Read the model definition and answer for the solid it produces. Units are mm, in the model's axes. Coordinates: 2 decimals unless noted, no trailing zeros. Write each loop counter-clockwise with the first axis right and the second up, starting at its lowest first coordinate (ties: lowest second). Pieces come first, ordered by that corner, then holes. Notation, with made-up numbers: (12, 7) -> (53, 7) arc R36 cw to (53, 44) -> close; hole circle Ø10 at (-2, 77). An arc over 180 degrees is marked (long way). Write item = value, one per line. Start each with the question number.
1) Flat-ended cylindrical pins translate along their axes: pin 1 Ø4 at (x, z) = (215.5, 6.5) entering from +Y; pin 2 Ø5 at (x, z) = (-51.5, 6) entering from -Y; pin 3 Ø4.5 at (y, z) = (-214, 5) entering from +X; pin 4 Ø5 at (x, z) = (-85, 9) entering from +Y. Find the tip coordinate at first contact, or state that the pin passes through.
2) Find the intervals of material crossed by line 1 along Y through (x, z) = (28, 5); line 2 along Y through (x, z) = (-43, 5.5), in increasing order. Write a range as from..to.
3) Section C-C (y = -120) is taken. Determine the outline of the cut face in (x, z), plus the area to 3 significant figures.
4) Section A-A (x = 87.5) is taken. Count the separate pieces of the cut face and the enclosed holes in it, plus the area to 3 significant figures.
from build123d import *

# Parameters (mm, degrees)
SKETCH_1_W             = 420
SKETCH_1_H             = 420
EXTRUDE_1_DEPTH        = 10
SKETCH_2_W             = 200
SKETCH_2_H             = 8
EXTRUDE_2_DEPTH        = 8
CUT_EXTRUDE_1_REACH    = 381.109
SKETCH_3_R             = 2
FILLET_1_R             = 4
FILLET_1_OF_MIRROR_1_R = 4
SKETCH_4_W             = 8
SKETCH_4_H             = 200
EXTRUDE_3_DEPTH        = 8
FILLET_2_R             = 4
CUT_EXTRUDE_2_REACH    = 387.679
SKETCH_5_R             = 2
FILLET_2_OF_MIRROR_3_R = 4


with BuildPart() as part:
    # 草图1 → 凸台-拉伸1 (new body)
    with BuildSketch(Plane.XY):
        Rectangle(SKETCH_1_W, SKETCH_1_H)
    extrude_1 = extrude(amount=EXTRUDE_1_DEPTH)

    # 草图2 → 凸台-拉伸2 (add)
    with BuildSketch(Plane(origin=(0, 210, 0), x_dir=(1, 0, 0), z_dir=(0, 1, 0))):
        with Locations((0, -5)):
            Rectangle(SKETCH_2_W, SKETCH_2_H)
    extrude_2 = extrude(amount=EXTRUDE_2_DEPTH)

    # 草图3 → 切除-拉伸1 (cut, up to next)
    with BuildSketch(Plane(origin=(100, 0, 0), x_dir=(0, 0, -1), z_dir=(1, 0, 0)), mode=Mode.PRIVATE) as cut_extrude_1_sk1:
        with Locations((-5, 214)):
            Circle(SKETCH_3_R)
    cut_extrude_1_tool1 = extrude(cut_extrude_1_sk1.sketch, amount=-CUT_EXTRUDE_1_REACH, mode=Mode.PRIVATE) & part.part
    cut_extrude_1 = cut_extrude_1_tool1.solids().sort_by_distance((100, 214, 5))[0]
    add(cut_extrude_1, mode=Mode.SUBTRACT)

    # 圆角1
    fillet_1_edges = [part.edges().sort_by_distance(p)[0] for p in [
        (0, 218, 1),
        (0, 218, 9),
    ]]
    fillet(fillet_1_edges, radius=FILLET_1_R - 0.0001)  # a hair under: the kernel refuses the full size

    # 镜向1: 凸台-拉伸1, 凸台-拉伸2, 切除-拉伸1 across plane
    add(extrude_1.mirror(Plane.ZX))
    add(extrude_2.mirror(Plane.ZX))
    add(cut_extrude_1.mirror(Plane.ZX), mode=Mode.SUBTRACT)

    # 圆角1 of 镜向1
    fillet_1_of_mirror_1_edges = [part.edges().sort_by_distance(p)[0] for p in [
        (0, -218, 1),
        (0, -218, 9),
    ]]
    fillet(fillet_1_of_mirror_1_edges, radius=FILLET_1_OF_MIRROR_1_R - 0.0001)  # a hair under: the kernel refuses the full size

    # 草图4 → 凸台-拉伸3 (add)
    with BuildSketch(Plane.ZY.offset(210)):
        with Locations((5, 0)):
            Rectangle(SKETCH_4_W, SKETCH_4_H)
    extrude_3 = extrude(amount=EXTRUDE_3_DEPTH)

    # 圆角2
    fillet_2_edges = [part.edges().sort_by_distance(p)[0] for p in [
        (-218, 0, 9),
        (-218, 0, 1),
    ]]
    fillet(fillet_2_edges, radius=FILLET_2_R - 0.0001)  # a hair under: the kernel refuses the full size

    # 草图5 → 切除-拉伸2 (cut, up to next)
    with BuildSketch(Plane.XZ.offset(100), mode=Mode.PRIVATE) as cut_extrude_2_sk1:
        with Locations(Location((-214, 5, 0), (0, 0, 270))):
            Circle(SKETCH_5_R)
    cut_extrude_2_tool1 = extrude(cut_extrude_2_sk1.sketch, amount=-CUT_EXTRUDE_2_REACH, mode=Mode.PRIVATE) & part.part
    cut_extrude_2 = cut_extrude_2_tool1.solids().sort_by_distance((-214, -100, 5))[0]
    add(cut_extrude_2, mode=Mode.SUBTRACT)

    # 镜向3: 凸台-拉伸3, 切除-拉伸2 across plane
    add(extrude_3.mirror(Plane(origin=(0, 0, 0), x_dir=(0, 0, 1), z_dir=(1, 0, 0))))
    add(cut_extrude_2.mirror(Plane(origin=(0, 0, 0), x_dir=(0, 0, 1), z_dir=(1, 0, 0))), mode=Mode.SUBTRACT)

    # 圆角2 of 镜向3
    fillet_2_of_mirror_3_edges = [part.edges().sort_by_distance(p)[0] for p in [
        (218, 0, 9),
        (218, 0, 1),
    ]]
    fillet(fillet_2_of_mirror_3_edges, radius=FILLET_2_OF_MIRROR_3_R - 0.0001)  # a hair under: the kernel refuses the full size


solid = part.part
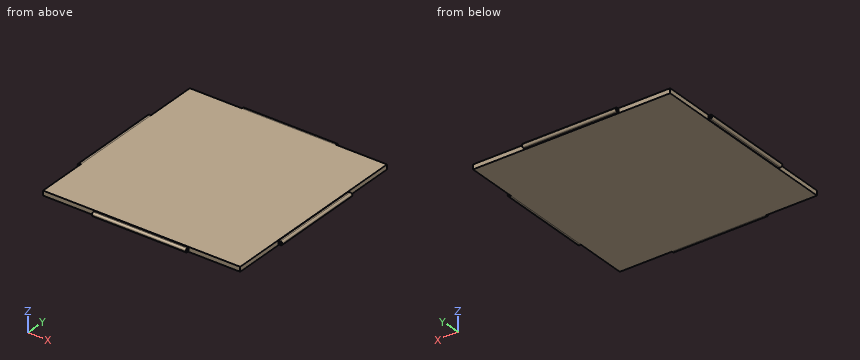
Answer key:
q1.pin_1 = 100
q1.pin_2 = -218
q1.pin_3 = 100
q1.pin_4 = 217.71
q2.line_1 = -218..-216, -212..212, 216..218
q2.line_2 = -217.97..-215.94, -212.06..212.06, 215.94..217.97
q3.outline = (-210, 0) -> (210, 0) -> (210, 10) -> (-210, 10) -> close
q3.area = 4,200 mm^2
q4.separate_pieces = 1
q4.enclosed_holes = 2
q4.area = 4,290 mm^2
